Verification items for this drawing (mm, ordinates from the low corner). A direction names the side the tool comes from. Round coordinates to 2 decimals unless told otherwise and drop trailing zeros. Order: outer loops, then holes, each group sorted by start corner. A loop starts at its lowest first (then second) coordinate and runs counter-clockwise, first axis right, second up. Notation, with made-up numbers: M 80,48 L 88,48 A24 ccw 88,76 Z; hole C 50.25,63 d7. An arc over 180 degrees is marked long. One line per item, written item: value. Start each with the question number.
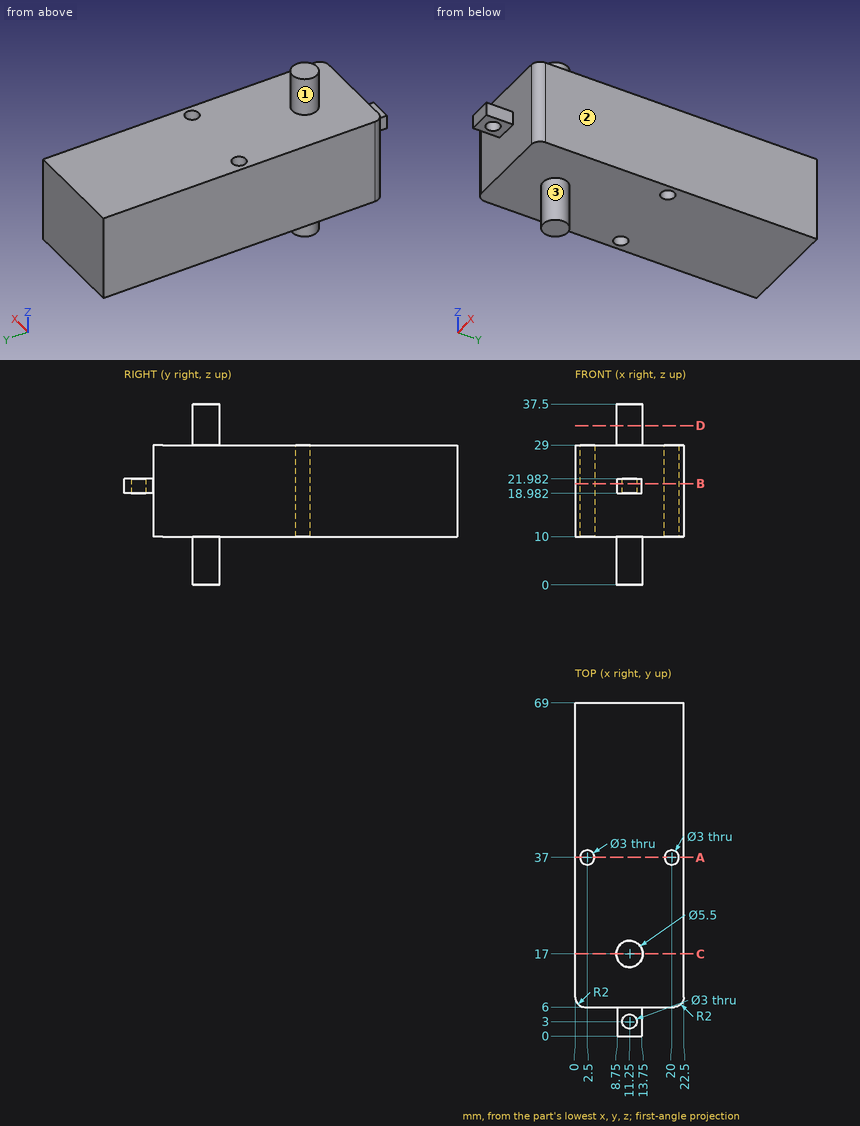
1. Scan lines: line 1 along Y through (x, z) = (20, 18.25); line 2 along Y through (x, z) = (11.25, 20.9); line 3 along Y through (x, z) = (16.5, 16.5). Record each from-to range of solid material in increasing order.
2. Tool access check on the marked faces 1, 2 and 3. Record the directions out of +Z, -Z, +X, -X, +Y, -Y that give a thin tool (end or side, any length) a straight path to the whole face; none if there is none.
3. Section check C-C (y = 17). Record the cut outline in (x, z).
4. Section check A-A (y = 37). Record the cut outline in (x, z).
5. Section check B-B (z = 21). Record the cut outline in (x, y), and give its area (3 significant figures).
6. Section check D-D (z = 33). Record the cut outline in (x, y).
7. Depth check by flat-ended pin: pin 1 (2 mm diameter, centred on x = 7.5, y = 13.5, fed in from -Z); pin 2 (12 mm diameter, centred on y = 29, z = 5.5, fed in from -X); pin 3 (3.5 mm diameter, centred on x = 2.5, y = 37, fed in from +Z); pin 4 (5 mm diameter, centred on x = 11.25, y = 3, fed in from +Z). Enter the tip coordinate at first touch or a pass-through.
Geometry check:
1. line 1: y = 6 to 35.5, 38.5 to 69
1. line 2: y = 0 to 1.5, 4.5 to 69
1. line 3: y = 6 to 69
2. face 1: +Z
2. face 2: +Z, -Z, +X, +Y, -Y
2. face 3: -Z
3. outline: M 0,10 L 8.5,10 L 8.5,0 L 14,0 L 14,10 L 22.5,10 L 22.5,29 L 14,29 L 14,37.5 L 8.5,37.5 L 8.5,29 L 0,29 Z
4. outline: M 0,10 L 1,10 L 1,29 L 0,29 Z; M 4,10 L 18.5,10 L 18.5,29 L 4,29 Z; M 21.5,10 L 22.5,10 L 22.5,29 L 21.5,29 Z
5. outline: M 0,8 A2 ccw 2,6 L 8.75,6 L 8.75,0 L 13.75,0 L 13.75,6 L 20.5,6 A2 ccw 22.5,8 L 22.5,69 L 0,69 Z; hole C 2.5,37 d3; hole C 11.25,3 d3; hole C 20,37 d3
5. area: 1,420 mm²
6. outline: C 11.25,17 d5.5
7. pin 1: stops at z = 10
7. pin 2: stops at x = 0
7. pin 3: stops at z = 29
7. pin 4: stops at z = 21.98
